from build123d import *

# Parameters (mm, degrees)
F0_W     = 40
F0_H     = 40
F0_W_2   = 33
F0_H_2   = 33
F1_DEPTH = 25
F2_W     = 40
F2_H     = 40
F3_DEPTH = 2
F4_W     = 5
F4_H     = 5
F5_DEPTH = 2
F6_W     = 18
F6_H     = 3.5
F7_DEPTH = 7
F8_R     = 5


with BuildPart() as f1:
    # F0 (on Top) → F1 (new body)
    with BuildSketch(Plane.XY):
        Rectangle(F0_W, F0_H)
        Rectangle(F0_W_2, F0_H_2, mode=Mode.SUBTRACT)
    extrude(amount=F1_DEPTH)

    # F2 (on Top) → F3 (join)
    with BuildSketch(Plane.XY):
        Rectangle(F2_W, F2_H)
    extrude(amount=-F3_DEPTH)

    # F4 (on face) → F5 (join)
    with BuildSketch(Plane.XY):
        with Locations((-14, 14)):
            Rectangle(F4_W, F4_H)
        with Locations((14, 14)):
            Rectangle(F4_W, F4_H)
        with Locations((-14, -14)):
            Rectangle(F4_W, F4_H)
        with Locations((14, -14)):
            Rectangle(F4_W, F4_H)
    extrude(amount=F5_DEPTH)

    # F6 (on face) → F7 (cut)
    with BuildSketch(Plane.XY):
        with Locations((0, -18.25)):
            Rectangle(F6_W, F6_H)
        with Locations((0, 18.25)):
            Rectangle(F6_W, F6_H)
    extrude(amount=F7_DEPTH, mode=Mode.SUBTRACT)

    # F8
    f8_edges = [f1.edges().sort_by_distance(p)[0] for p in [
        (20, -20, 11.5),
        (-20, -20, 11.5),
        (20, 20, 11.5),
        (-20, 20, 11.5),
    ]]
    fillet(f8_edges, radius=F8_R)


solid = f1.part
Design review of the part built by this model. Coordinates are the model's own, in mm. A direction names the side the tool comes from. Give positions to 0.01 mm unless a question says otherwise; leave off trailing zeros. Loops run counter-clockwise (first coordinate to the right, second up) from the corner with the lowest first, then second, coordinate; pieces in that order, holes last. Notation, with made-up numbers: (-36.5, 57.25) - (5.5, 57.25) arc R21 ccw to (5.5, 82.25) - close; hole circle Ø10 at (25, -17). An arc over 180 degrees is marked (long way). Write item = value, one per line.
1) Take a section at B-B on z = 13.75. State the section outline as (x, y) points, and give its area (3 significant figures).
Result sheet:
outline = (-20, -15) arc R5 ccw to (-15, -20) - (15, -20) arc R5 ccw to (20, -15) - (20, 15) arc R5 ccw to (15, 20) - (-15, 20) arc R5 ccw to (-20, 15) - close; hole (-16.5, -16.5) - (16.5, -16.5) - (16.5, 16.5) - (-16.5, 16.5) - close
area = 490 mm2
2) Clearance check with flat-ended pins moving along their axes: pin 1 Ø1.5 at (x, y) = (-14.5, 13.5) entering from +Z; pin 2 Ø5 at (x, y) = (8.5, 12) entering from +Z; pin 3 Ø1 at (y, z) = (18, 4) entering from +X. State where each tip first meets the part, or that it passes through.
Result sheet:
pin_1 = 2
pin_2 = 0
pin_3 = 19.33
3) Take a section at A-A on x = -4.5. State the section outline as (y, z) points.
Result sheet:
outline = (-20, -2) - (20, -2) - (20, 0) - (-20, 0) - close; (-20, 7) - (-16.5, 7) - (-16.5, 25) - (-20, 25) - close; (16.5, 7) - (20, 7) - (20, 25) - (16.5, 25) - close
4) Take a section at C-C on y = -3.5. State the section outline as (x, z) points.
Result sheet:
outline = (-20, -2) - (20, -2) - (20, 25) - (16.5, 25) - (16.5, 0) - (-16.5, 0) - (-16.5, 25) - (-20, 25) - close
5) Draft analysis for pull direction Z (two halves, no side actions). For faces 4 (the face through (0, 18, 7)), 5 (the face through (-14, -14, 2)), 6 (the face through (11.5, -14, 1)), state which applies: +Z half, -Z half, draft (parallel to the pull), parting line (faces both ways), or undercut.
Result sheet:
face_4 = undercut
face_5 = +Z half
face_6 = draft
6) To check wall thickness, follow line 1 (X direction, y = -3, z = 19); line 2 (Z direction, x = 15, y = -5). State the ranges of each line that lie inside material, in increasing order.
Result sheet:
line_1 = -20 to -16.5, 16.5 to 20
line_2 = -2 to 0
7) Tool access review of faces 1 (the face through (9, -18, 3)), 2 (the face through (14, -14, 2)), 3 (the face through (0, 20, 12)): name each direction out of +Z, -Z, +X, -X, +Y, -Y from which nothing blocks a thin tool from reaching the whole face with its end or side.
Result sheet:
face_1 = +Y, -Y
face_2 = +Z
face_3 = +Z, -Z, +X, -X, +Y
